from build123d import *

# Parameters (mm, degrees)
F2_R     = 3.8735
F3_DEPTH = 41.276
F5_DEPTH = 3.175


with BuildPart() as f1:
    # F0 (on Front) → F1 (revolve)
    with BuildSketch(Plane.XZ):
        Polygon((-24.384, 38.1), (-25.4, 38.1), (-44.45, 0), (0, 0), (0, 41.275), (-5.461, 41.275), (-5.461, 38.1), (-7.874, 38.1), (-5.461, 34.653879), (-5.461, 3.175), (-35.762984, 3.175), (-18.300484, 38.1), (-20.828, 38.1), (-21.336, 37.592), (-21.336, 35.56), (-23.876, 35.56), (-23.876, 37.592), align=None)
    revolve(axis=Axis((0, 0, 21.25227), (0, 0, 1)))

    # F2 (on face) → F3 (cut, through all)
    with BuildSketch(Plane.XY.offset(41.275)):
        Circle(F2_R)
    extrude(amount=-F3_DEPTH, mode=Mode.SUBTRACT)

    # F4 (on face) → F5 (cut)
    with BuildSketch(Plane(origin=(0, 0, 0), x_dir=(1, 0, 0), z_dir=(0, 0, -1))):
        with BuildLine():
            ThreePointArc((-6.210474, 1.323825), (-5.399143, 3.342418), (-3.954071, 4.968684))
            ThreePointArc((-3.954071, 4.968684), (-3.20282, 5.829119), (-2.804688, 6.899734))
            ThreePointArc((-2.804688, 6.899734), (2.007902, 17.190565), (11.32741, 23.687409))
            ThreePointArc((11.32741, 23.687409), (13.423957, 26.641414), (11.387913, 29.637442))
            ThreePointArc((11.387913, 29.637442), (-10.902012, 29.819601), (-27.818336, 15.303682))
            ThreePointArc((-27.818336, 15.303682), (-28.138147, 14.451862), (-28.203233, 13.544315))
            ThreePointArc((-28.203233, 13.544315), (-21.766814, 1.757015), (-8.648102, -1.11828))
            ThreePointArc((-8.648102, -1.11828), (-7.068588, -0.257266), (-6.210474, 1.323825))
        make_face()
        with BuildLine():
            ThreePointArc((1.958771, -6.040341), (-0.195047, -6.347004), (-2.325971, -5.908668))
            ThreePointArc((-2.325971, -5.908668), (-3.446755, -5.688283), (-4.573001, -5.878798))
            ThreePointArc((-4.573001, -5.878798), (-15.891416, -6.856388), (-26.177603, -2.03388))
            ThreePointArc((-26.177603, -2.03388), (-29.78412, -1.695219), (-31.360734, -4.956499))
            ThreePointArc((-31.360734, -4.956499), (-20.373526, -24.35122), (0.655791, -31.743227))
            ThreePointArc((0.655791, -31.743227), (1.553394, -31.594281), (2.371896, -31.196874))
            ThreePointArc((2.371896, -31.196874), (9.361787, -19.729122), (5.29251, -6.930337))
            ThreePointArc((5.29251, -6.930337), (3.757093, -5.992944), (1.958771, -6.040341))
        make_face()
        with BuildLine():
            ThreePointArc((4.251703, 4.716516), (5.59419, 3.004586), (6.280042, 0.939984))
            ThreePointArc((6.280042, 0.939984), (6.649575, -0.140836), (7.377689, -1.020936))
            ThreePointArc((7.377689, -1.020936), (13.883515, -10.334176), (14.850193, -21.653529))
            ThreePointArc((14.850193, -21.653529), (16.360163, -24.946195), (19.972821, -24.680942))
            ThreePointArc((19.972821, -24.680942), (31.275538, -5.468381), (27.162545, 16.439545))
            ThreePointArc((27.162545, 16.439545), (26.584753, 17.142419), (25.831337, 17.652559))
            ThreePointArc((25.831337, 17.652559), (12.405027, 17.972106), (3.355593, 8.048616))
            ThreePointArc((3.355593, 8.048616), (3.311495, 6.25021), (4.251703, 4.716516))
        make_face()
    extrude(amount=-F5_DEPTH, mode=Mode.SUBTRACT)


solid = f1.part
Geometry: final body of the model. Coordinates: model frame, mm. A direction names the side the tool comes from. Coordinates: 2 decimals unless noted, no trailing zeros.
1) Section A-A (x = -15). Give the number of separate pieces and of enclosed holes in the cut face, then the cut area to 3 significant figures.
Result sheet:
separate pieces: 3
enclosed holes: 0
area: 667 mm2
2) Set-up query: faces 4 (the cylindrical face through (13.423, -26.587, 1.565)), 5 (the cylindrical face through (5.176, 23.308, 36.59)), 6 (the flat face through (1, -11, 0)), 7 (the cylindrical face through (-5.21, -1.64, 18.69)), 8 (the cylindrical face through (2.08, 3.27, 20.93)). Return all of +Z, -Z, +X, -X, +Y, -Y with unobstructed straight access to the full face (end or side cutting, diameter ignored); none if empty.
Result sheet:
face 4: -Z
face 5: +Z
face 6: -Z, +X, -X, +Y, -Y
face 7: none
face 8: +Z, -Z
3) Draft query along Z for faces 1 (the flat face through (2.5, -5.5, 3.175)), 2 (the flat face through (-10, -23, 38.1)), 3 (the cylindrical face through (-3.43, 5.69, 1.57)). Return one class per face: released by +Z, released by -Z, zero draft, split by the parting line, or undercut.
Result sheet:
face 1: undercut
face 2: released by +Z
face 3: zero draft
4) First-contact query: P1, Ø3, axis at x = 0, z = 6, coming from the -Y side; P2, Ø12, axis at x = -12, y = 20.5, coming from the +Z side; P3, Ø2, axis at x = -11, z = 17, coming from the +Y side; P4, Ø4.5, axis at x = 0, y = 0, coming from the -Z side. Flat tips, straight axial feed; report the tip coordinate or a pass-through.
Result sheet:
P1: stops at y = -42.2
P2: stops at z = 38.1
P3: stops at y = 34.83
P4: passes through
5) Ray query, probe 1 along Y at (x, z) = (0, 31.5); probe 2 along Y at (x, z) = (0, 21.5); probe 3 along Y at (x, z) = (0, 37.15) (1 decimal). Return the intervals inside material, ascending.
Result sheet:
probe 1: y = -28.7 to -21.6, -5.46 to -3.87, 3.87 to 5.46, 21.6 to 28.7
probe 2: y = -33.7 to -26.6, -5.46 to -3.87, 3.87 to 5.46, 26.6 to 33.7
probe 3: y = -25.9 to -23.9, -21.3 to -18.8, -7.2 to -3.9, 3.9 to 7.2, 18.8 to 21.3, 23.9 to 25.9
